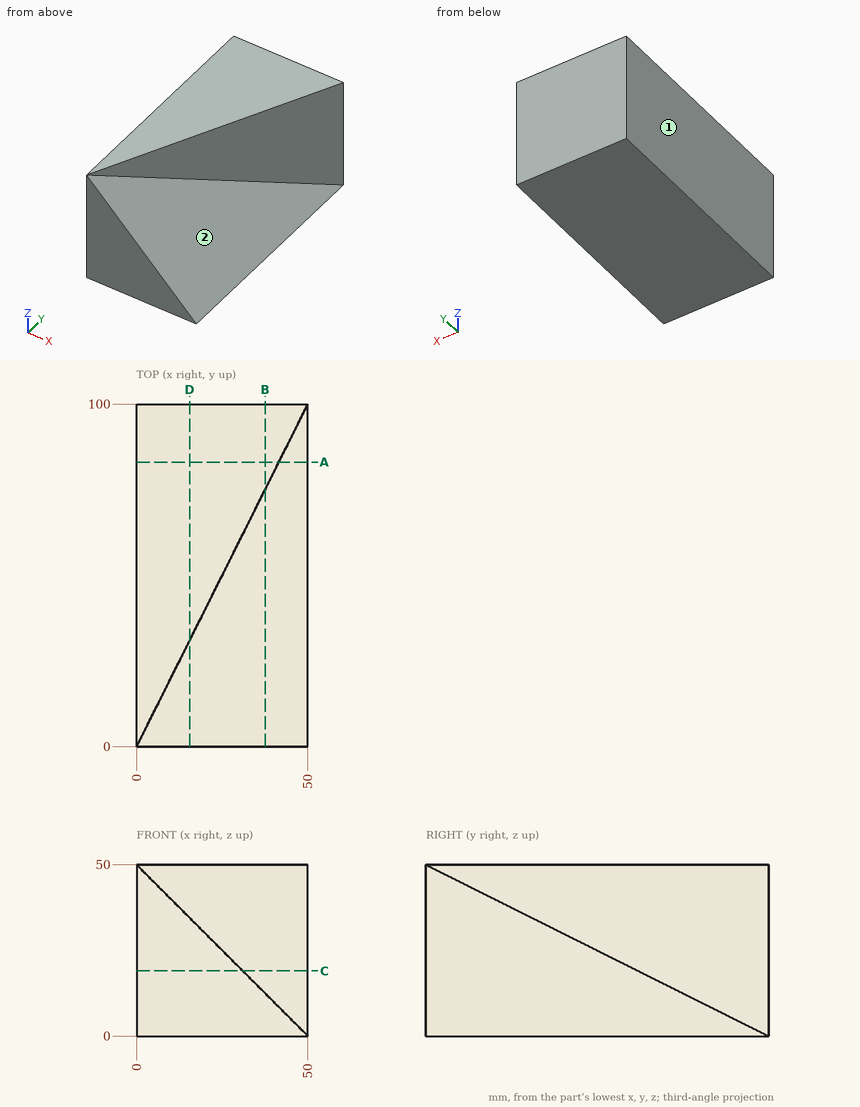
Job drawing, mm, ordinate dimensions from the low corner. One solid piece. A direction names the side the tool comes from. Give positions to 0.01 mm unless a question says otherwise; leave off trailing zeros. Order: outer loops, then holes, each group sorted by start corner. A loop starts at its lowest first (then second) coordinate and runs counter-clockwise, first axis right, second up. Notation, with made-up numbers: M 17.5,85 L 60.5,85 A24 ccw 60.5,112 Z; hole C 63,21.25 d3. An arc over 180 degrees is marked long. Put each result on its own line as item: value. Start each with the question number.
(1) Band-saw the part on C-C on z = 19. Give the cut face in (x, y).
(2) Band-saw the part on D-D on x = 15.5. Give the cut face in (y, z).
(3) Pin check, flat tips, straight feed: pin 1 Ø12 at (x, y) = (23.5, 47) entering from -Z; pin 2 Ø12 at (x, y) = (30.5, 39) entering from +Z. Stop position of each tip, or through.
(4) Band-saw the part on A-A on y = 83. Give the cut face in (x, z), then the cut area to 3 significant figures.
(5) Drill centre lines: L1, parallel to X at y = 32, z = 12; L2, parallel to Z at x = 26, y = 42; L3, parallel to X at y = 74, z = 6. Where is each one in solid material? Low to high. Write a range as [from, to].
(6) Band-saw the part on B-B on x = 37.5. Give the cut face in (y, z), then the cut area to 3 significant figures.
(7) Tool access for the marked faces 1 and 2: list every direction of +Z, -Z, +X, -X, +Y, -Y with a clear straight run to the whole face (end or side of a thin tool).
Results below:
1. outline: M 0,0 L 31,0 L 31,62 L 50,100 L 0,100 Z
2. outline: M 0,0 L 100,0 L 100,50 L 31,50 L 31,34.5 L 0,34.5 Z
3. pin 1: stops at z = 0
3. pin 2: stops at z = 25.5
4. outline: M 0,0 L 50,0 L 41.5,8.5 L 41.5,50 L 0,50 Z
4. area: 2,110 mm2
5. L1: x = [0, 38]
5. L2: z = [0, 24]
5. L3: x = [0, 44]
6. outline: M 0,0 L 100,0 L 100,50 L 75,50 L 75,12.5 L 0,12.5 Z
6. area: 2,190 mm2
7. face 1: +Z, -Z, -X, +Y, -Y
7. face 2: +Z, +X, -Y
